from build123d import *

# Parameters (mm, degrees)
SKETCH_W        = 130
SKETCH_H        = 200
PAD_DEPTH       = 2.5
SKETCH001_R     = 2.5
POCKET_DEPTH    = 5.001
SKETCH002_R     = 19
SKETCH002_R_2   = 2.5
POCKET001_DEPTH = 5.001


with BuildPart() as part:
    # Sketch → Pad (new body, symmetric)
    with BuildSketch(Plane.YZ):
        Rectangle(SKETCH_W, SKETCH_H)
    extrude(amount=PAD_DEPTH, both=True)

    # Sketch001 (on Face6 of Pad) → Pocket (cut, through all)
    with BuildSketch(Plane.YZ.offset(2.5)):
        with Locations((-50, 85)):
            Circle(SKETCH001_R)
        with Locations((45, 85)):
            Circle(SKETCH001_R)
        with Locations((-50, -85)):
            Circle(SKETCH001_R)
        with Locations((45, -85)):
            Circle(SKETCH001_R)
    extrude(amount=-POCKET_DEPTH, mode=Mode.SUBTRACT)

    # Sketch002 (on Face5 of Pocket) → Pocket001 (cut, through all)
    with BuildSketch(Plane.YZ.offset(2.5)):
        with Locations((0, 66)):
            Circle(SKETCH002_R)
        with Locations((-16, 82)):
            Circle(SKETCH002_R_2)
        with Locations((16, 82)):
            Circle(SKETCH002_R_2)
        with Locations((16, 50)):
            Circle(SKETCH002_R_2)
        with Locations((-16, 50)):
            Circle(SKETCH002_R_2)
    extrude(amount=-POCKET001_DEPTH, mode=Mode.SUBTRACT)


solid = part.part
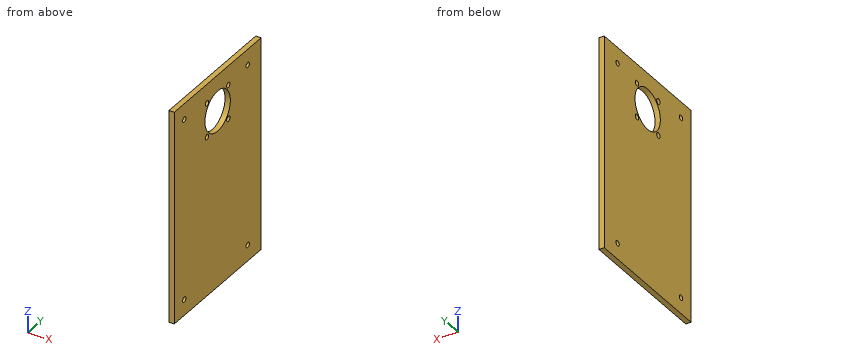
Geometry check sheet. Reference: the model listing, model coordinates, mm. Give positions to 0.01 mm unless a question says otherwise; leave off trailing zeros. Loops run counter-clockwise (first coordinate to the right, second up) from the corner with the lowest first, then second, coordinate; pieces in that order, holes last.
(1) Section check C-C on z = 66. Record the cut outline in (x, y).
From the geometry:
outline: (-2.5, -65) - (2.5, -65) - (2.5, -19) - (-2.5, -19) - close; (-2.5, 19) - (2.5, 19) - (2.5, 65) - (-2.5, 65) - close
(2) Section check D-D on x = -1.4. Count the separate pieces of the cut face and the enclosed holes in it, then the cut area to 3 significant figures.
From the geometry:
separate pieces: 1
enclosed holes: 9
area: 24,700 mm2
(3) Depth check by flat-ended pin: pin 1 Ø4.5 at (y, z) = (-50, -85) entering from +X. Enter the tip coordinate at first touch or a pass-through.
From the geometry:
pin 1: passes through
(4) Thickness scan on L1, parallel to Z at x = -1.25, y = -50; L2, parallel to Z at x = -1.35, y = -16; L3, parallel to Y at x = 2.2, z = 70.5. Record the ranges inside material, lowest first.
From the geometry:
L1: z = -100 to -87.5, -82.5 to 82.5, 87.5 to 100
L2: z = -100 to 47.5, 52.5 to 55.75, 76.25 to 79.5, 84.5 to 100
L3: y = -65 to -18.46, 18.46 to 65
(5) Section check B-B on y = 45. Record the cut outline in (x, z), then the cut area to 3 significant figures.
From the geometry:
outline: (-2.5, -100) - (2.5, -100) - (2.5, -87.5) - (-2.5, -87.5) - close; (-2.5, -82.5) - (2.5, -82.5) - (2.5, 82.5) - (-2.5, 82.5) - close; (-2.5, 87.5) - (2.5, 87.5) - (2.5, 100) - (-2.5, 100) - close
area: 950 mm2
(6) Section check A-A on y = 0. Record the cut outline in (x, z).
From the geometry:
outline: (-2.5, -100) - (2.5, -100) - (2.5, 47) - (-2.5, 47) - close; (-2.5, 85) - (2.5, 85) - (2.5, 100) - (-2.5, 100) - close
